Autodesk Inventor part; units mm, degrees
ref_plane "YZ Plane" through (0, 0, 0) normal (1, 0, 0) x (0, 1, 0)
ref_plane "XZ Plane" through (0, 0, 0) normal (0, 1, 0) x (-1, 0, 0)
ref_plane "XY Plane" through (0, 0, 0) normal (0, 0, 1) x (1, 0, 0)
sketch "Sketch1" plane through (0, 0, 0) normal (1, 0, 0) x (0, 1, 0)
  line L0 (0, 0) -> (50.8, 0)
  line L1 (50.8, 0) -> (50.8, -25.4)
  line L2 (50.8, -25.4) -> (0, -25.4)
  line L3 (0, -25.4) -> (0, 0)
  line L4 (49.53, -1.27) -> (1.27, -1.27)
  line L5 (1.27, -1.27) -> (1.27, -24.13)
  line L6 (1.27, -24.13) -> (49.53, -24.13)
  line L7 (49.53, -24.13) -> (49.53, -1.27)
  dimension "d0" = 50.8
  dimension "d1" = 25.4
  dimension "d2" = 1.27
extrude "Extrusion1" add sketch "Sketch1" along normal blind 279.4
sketch "Sketch2" plane through (0, 0, 0) normal (0, 0, 1) x (1, 0, 0)
  circle A0 centre (246.6677, 25.4) radius 7.3323
  point P0 (0, 0)
extrude "Extrusion2" cut sketch "Sketch2" against normal through all
sketch "Sketch3" plane through (279.4, 49.53, -1.27) normal (0, 0, -1) x (-1, 0, 0)
  circle A0 centre (8.9208, -23.9155) radius 2.5908
  circle A1 centre (21.0377, -3.4163) radius 2.5908
  circle A2 centre (20.6153, -44.6586) radius 2.5908
  circle A3 centre (56.5433, -24.4032) radius 2.5908
  circle A4 centre (44.4265, -44.9024) radius 2.5908
  circle A5 centre (44.8489, -3.6601) radius 2.5908
  point P0 (279.4, -49.53)
extrude "Extrusion3" cut sketch "Sketch3" along normal through all both and the other way through all
properties part number "Aluminum grabber mount"
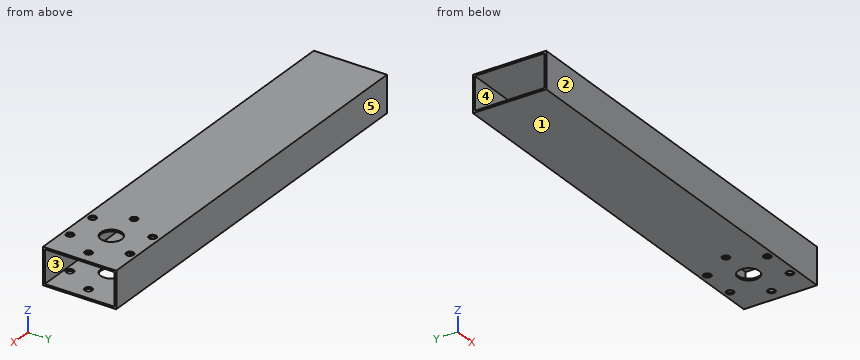
CAD build for the part. Positions are in the model's coordinates, mm. Face numbers are marked on the shaded views. A direction names the side the tool comes from. Round coordinates to 2 decimals unless told otherwise and drop trailing zeros. Write each loop counter-clockwise with the first axis right and the second up, starting at its lowest first coordinate (ties: lowest second). Pieces come first, ordered by that corner, then holes.
Item 1: Band-saw the part on B-B on y = 39.5. Write the cut outline in (x, z), then the cut area to 3 significant figures.
Filled in:
outline: (0, -25.4) - (279.4, -25.4) - (279.4, -24.13) - (0, -24.13) - close; (0, -1.27) - (279.4, -1.27) - (279.4, 0) - (0, 0) - close
area: 710 mm2
Item 2: Band-saw the part on A-A on z = -11.5. Write the cut outline in (x, y).
Filled in:
outline: (0, 0) - (279.4, 0) - (279.4, 1.27) - (0, 1.27) - close; (0, 49.53) - (279.4, 49.53) - (279.4, 50.8) - (0, 50.8) - close
Item 3: Tool access for the marked faces 4 and 5: list every direction of +Z, -Z, +X, -X, +Y, -Y with a clear straight run to the whole face (end or side of a thin tool).
Filled in:
face 4: +X, -X
face 5: +Z, -Z, +X, -X, +Y
Item 4: Mould opens along Y. For the marked faces 1, 2 and 3 say: released by +Y, released by -Y, zero draft, split by the parting line, or undercut.
Filled in:
face 1: zero draft
face 2: released by -Y
face 3: undercut
Item 5: Band-saw the part on C-C on x = 136.5. Write the cut outline in (y, z), then the cut area to 3 significant figures.
Filled in:
outline: (0, -25.4) - (50.8, -25.4) - (50.8, 0) - (0, 0) - close; hole (1.27, -24.13) - (49.53, -24.13) - (49.53, -1.27) - (1.27, -1.27) - close
area: 187 mm2
Item 6: Drill centre lines: L1, parallel to Y at x = 52, z = -7.5; L2, parallel to Z at x = 81.5, y = 3. Where is each one in solid material? Low to high.
Filled in:
L1: y = 0 to 1.27, 49.53 to 50.8
L2: z = -25.4 to -24.13, -1.27 to 0
